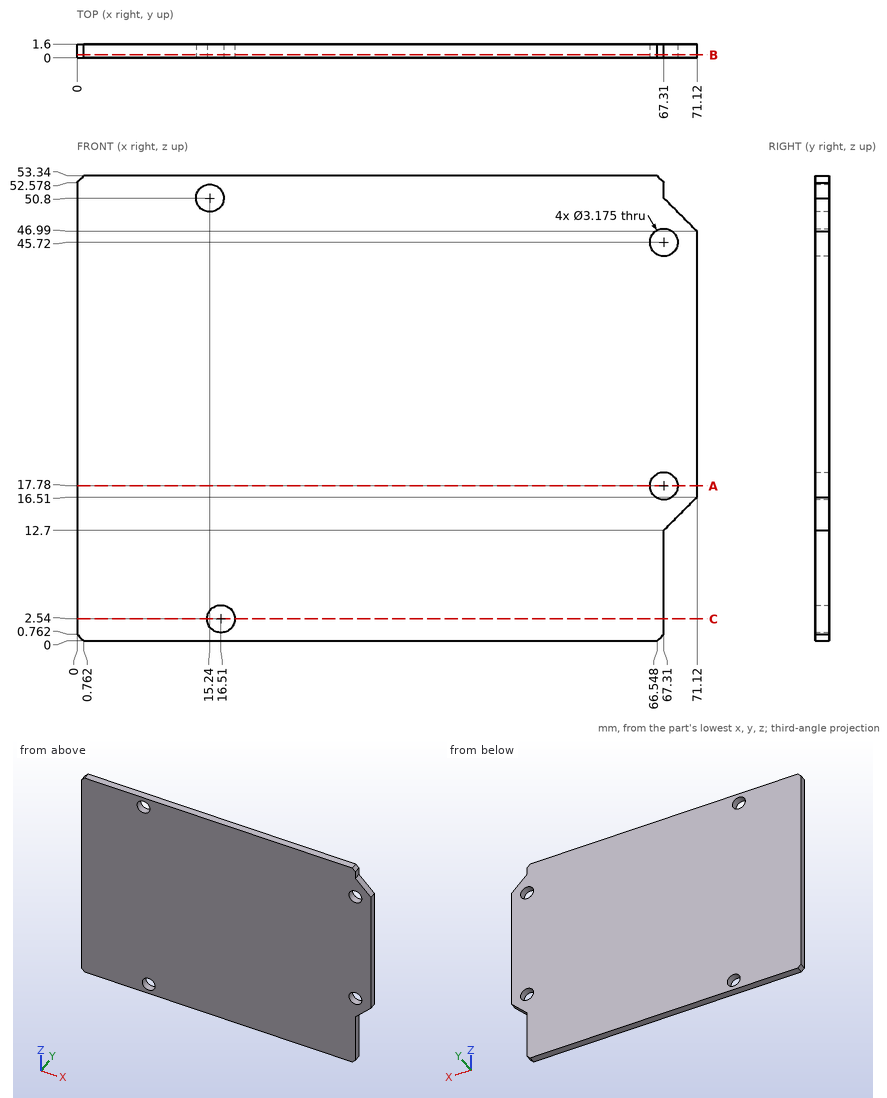
For this review, use the dimensioned drawing (mm, ordinates from the lowest corner) and the shaded views. Round coordinates to 2 decimals unless told otherwise and drop trailing zeros. Order: outer loops, then holes, each group sorted by start corner. A loop starts at its lowest first (then second) coordinate and runs counter-clockwise, first axis right, second up. Notation, with made-up numbers: (47, 27) -> (61, 27) arc R20 ccw to (61, 61) -> close; hole circle Ø3 at (13, 22.25). An arc over 180 degrees is marked (long way). One line per item, written item: value. Start each with the question number.
Q1. Take a section at C-C (z = 2.54). Write out the cut boundary in (x, y), and give its area (3 significant figures).
Q2. Wall thickness on line 1 (X direction, y = 0.6, z = 2.54); line 2 (X direction, y = 0.85, z = 17.78); line 3 (X direction, y = 0.9, z = 9.5): over which ranges is each line inside the solid? List them lowest first.
Q3. Clearance check with flat-ended pins moving along their axes: pin 1 Ø1.9 at (x, z) = (15.24, 50.8) entering from -Y; pin 2 Ø0.8 at (y, z) = (1, 7.5) entering from +X. State where each tip first meets the part, or that it passes through.
Q4. Take a section at A-A (z = 17.78). Write out the cut boundary in (x, y).
Q5. Take a section at B-B (y = 0.35). Write out the cut boundary in (x, z) (1 decimal).
Reported:
1. outline: (0, 0) -> (14.92, 0) -> (14.92, 1.6) -> (0, 1.6) -> close; (18.1, 0) -> (67.31, 0) -> (67.31, 1.6) -> (18.1, 1.6) -> close
1. area: 103 mm2
2. line 1: x = 0 to 14.92, 18.1 to 67.31
2. line 2: x = 0 to 65.72, 68.9 to 71.12
2. line 3: x = 0 to 67.31
3. pin 1: passes through
3. pin 2: stops at x = 67.31
4. outline: (0, 0) -> (65.72, 0) -> (65.72, 1.6) -> (0, 1.6) -> close; (68.9, 0) -> (71.12, 0) -> (71.12, 1.6) -> (68.9, 1.6) -> close
5. outline: (0, 0.8) -> (0.8, 0) -> (66.5, 0) -> (67.3, 0.8) -> (67.3, 12.7) -> (71.1, 16.5) -> (71.1, 47) -> (67.3, 50.8) -> (67.3, 52.6) -> (66.5, 53.3) -> (0.8, 53.3) -> (0, 52.6) -> close; hole circle Ø3.2 at (15.2, 50.8); hole circle Ø3.2 at (16.5, 2.5); hole circle Ø3.2 at (67.3, 17.8); hole circle Ø3.2 at (67.3, 45.7)
